from build123d import *

# Parameters (mm, degrees)
F1_DEPTH = 15.7734
F2_R     = 28.575
F3_DEPTH = 40.2336
F4_R     = 3.302


with BuildPart() as f1:
    # F0 (on Top) → F1 (new body)
    with BuildSketch(Plane.XY):
        with BuildLine():
            ThreePointArc((28.575, 0), (23.3274655355, -16.5033322905), (9.5121844836, -26.9452959039))
            Line((9.5121844836, -26.9452959039), (57.1919272622, -18.7764181619))
            ThreePointArc((57.1919272622, -18.7764181619), (73.025, 0), (57.1919272622, 18.7764181619))
            Line((57.1919272622, 18.7764181619), (9.5121844836, 26.9452959039))
            ThreePointArc((9.5121844836, 26.9452959039), (23.3274655355, 16.5033322905), (28.575, 0))
        make_face()
        with BuildLine():
            ThreePointArc((64.135, 0), (53.975, -10.16), (43.815, 0))
            ThreePointArc((43.815, 0), (53.975, 10.16), (64.135, 0))
        make_face(mode=Mode.SUBTRACT)
    extrude(amount=F1_DEPTH)

    # F2 (on Top) → F3 (join)
    with BuildSketch(Plane.XY):
        Circle(F2_R)
        with BuildLine():
            ThreePointArc((13.4477648793, -4.826), (-14.2874992271, 0.0046994463), (13.4509367064, 4.8171524752))
            Line((13.4509367064, 4.8171524752), (18.5293, 4.8171524752))
            Line((18.5293, 4.8171524752), (18.5293, 0))
            Line((18.5293, 0), (18.5293, -4.826))
            Line((18.5293, -4.826), (13.4477648793, -4.826))
        make_face(mode=Mode.SUBTRACT)
    extrude(amount=F3_DEPTH)

    # F4
    f4_edges = [f1.edges().sort_by_distance(p)[0] for p in [
        (-28.575, 0, 40.2336),
    ]]
    fillet(f4_edges, radius=F4_R)


solid = f1.part
CAD build for the part. Positions are in the model's coordinates, mm. A direction names the side the tool comes from. Give positions to 0.01 mm unless a question says otherwise; leave off trailing zeros. Loops run counter-clockwise (first coordinate to the right, second up) from the corner with the lowest first, then second, coordinate; pieces in that order, holes last. Notation, with made-up numbers: M 14.5,53.5 L 46.5,53.5 A12 ccw 46.5,58.5 Z; hole C -38.75,39 d2. An arc over 180 degrees is marked long. One line per question, with ' | ' between items. Start each with the question number.
1. Saw through at A-A on y = 0. Give the cut face in (x, z) (1 decimal).
2. Probe L1, parallel to Y at x = 0, z = 9 (1 decimal); L2, parallel to X at y = 0, z = 20.5 (1 decimal); L3, parallel to Y at x = 3, z = 17. List the from-to ranges inside material, lowest first. Write a range as from..to.
3. Saw through at B-B on x = 0. Give the cut face in (y, z) (1 decimal).
4. Saw through at D-D on z = 14. State how many separate pieces and enclosed holes the cut face has, plus the area to 3 significant figures.
5. 3-axis set-ups, long thin cutter, end or side, ignore diameter. For faces 4 (the face through (33.7, 22.8, 7.8)), 5 (the face through (18.529, 0, 20)): which of +Z, -Z, +X, -X, +Y, -Y reach the whole face in a straight line?
6. Two-plate mould, pull along X, no slides. Class faces 1 (the face through (-14.277, -0.555, 19.835)), 2 (the face through (-28.547, 1.256, 22.311)), 3 (the face through (73.02, -0.37, 7.78)): pulls with the +X half, pulls with the -X half, needs draft (parallel to the pull), parting line crosses it, or undercut.
7. Flat gauge pins, fed straight in: pin 1 (2 mm diameter, centred on x = 48.5, z = 5, fed in from +Y); pin 2 (4 mm diameter, centred on y = 15, z = 17, fed in from -X); pin 3 (1 mm diameter, centred on y = 9.5, z = 21.5, fed in from +X); pin 4 (3 mm diameter, centred on x = 62, z = 18.5, fed in from -Y). Where does each tip first touch, or does it go through?
Result sheet:
1) outline: M -28.6,0 L -14.3,0 L -14.3,40.2 L -25.3,40.2 A3.3 ccw -28.6,36.9 Z; M 18.5,0 L 43.8,0 L 43.8,15.8 L 28.6,15.8 L 28.6,36.9 A3.3 ccw 25.3,40.2 L 18.5,40.2 Z; M 64.1,0 L 73,0 L 73,15.8 L 64.1,15.8 Z
2) L1: y = -28.6..-14.3, 14.3..28.6 | L2: x = -28.6..-14.3, 18.5..28.6 | L3: y = -28.42..-13.97, 13.97..28.42
3) outline: M -28.6,0 L -14.3,0 L -14.3,40.2 L -25.3,40.2 A3.3 ccw -28.6,36.9 Z; M 14.3,0 L 28.6,0 L 28.6,36.9 A3.3 ccw 25.3,40.2 L 14.3,40.2 Z
4) separate pieces: 1 | enclosed holes: 2 | area: 3,430 mm^2
5) face 4: +Z, -Z, +X, +Y | face 5: +Z, -Z
6) face 1: undercut | face 2: parting line crosses it | face 3: pulls with the +X half
7) pin 1: stops at y = 20.44 | pin 2: stops at x = -25.45 | pin 3: stops at x = 27.12 | pin 4: passes through
